```python
from build123d import *

# Parameters (mm, degrees)
SKETCH_W        = 54.3
SKETCH_H        = 39
PAD_DEPTH       = 2
SKETCH001_W     = 54.3
SKETCH001_H     = 2
PAD001_DEPTH    = 22
SKETCH003_W     = 6.85
SKETCH003_H     = 15
PAD003_DEPTH    = 22
SKETCH004_R     = 1.5
POCKET_DEPTH    = 15
SKETCH005_W     = 6.85
SKETCH005_H     = 15
PAD004_DEPTH    = 22
SKETCH006_R     = 1.5
POCKET001_DEPTH = 15
SKETCH007_W     = 25
SKETCH007_H     = 2
PAD005_DEPTH    = 22
POCKET002_DEPTH = 2.5
POCKET003_DEPTH = 5
FILLET_R        = 3
FILLET001_R     = 3
FILLET002_R     = 3
FILLET003_R     = 3
FILLET004_R     = 3
SKETCH010_R     = 1.786385
POCKET004_DEPTH = 5


with BuildPart() as part:
    # Sketch → Pad (new body)
    with BuildSketch(Plane.XY):
        with Locations((27.15, 21.5)):
            Rectangle(SKETCH_W, SKETCH_H)
    extrude(amount=PAD_DEPTH)

    # Sketch001 → Pad001 (join)
    with BuildSketch(Plane.XY):
        with Locations((27.15, 1)):
            Rectangle(SKETCH001_W, SKETCH001_H)
    extrude(amount=PAD001_DEPTH)

    # Sketch003 → Pad003 (join)
    with BuildSketch(Plane.XY):
        with Locations((3.425, 20.3)):
            Rectangle(SKETCH003_W, SKETCH003_H)
    extrude(amount=PAD003_DEPTH)

    # Sketch004 (on Face14 of Pad003) → Pocket (cut)
    with BuildSketch(Plane(origin=(0, 27.8, 0), x_dir=(-1, 0, 0), z_dir=(0, 1, 0))):
        with Locations((-3, 17)):
            Circle(SKETCH004_R)
        with Locations((-3, 7)):
            Circle(SKETCH004_R)
    extrude(amount=-POCKET_DEPTH, mode=Mode.SUBTRACT)

    # Sketch005 → Pad004 (join)
    with BuildSketch(Plane.XY):
        with Locations((50.875, 20.3)):
            Rectangle(SKETCH005_W, SKETCH005_H)
    extrude(amount=PAD004_DEPTH)

    # Sketch006 (on Face13 of Pad004) → Pocket001 (cut)
    with BuildSketch(Plane(origin=(0, 27.8, 0), x_dir=(-1, 0, 0), z_dir=(0, 1, 0))):
        with Locations((-51.3, 17)):
            Circle(SKETCH006_R)
        with Locations((-51.3, 7)):
            Circle(SKETCH006_R)
    extrude(amount=-POCKET001_DEPTH, mode=Mode.SUBTRACT)

    # Sketch007 (on Face4 of Pocket001) → Pad005 (join)
    with BuildSketch(Plane(origin=(0, 0, 0), x_dir=(1, 0, 0), z_dir=(0, 0, -1))):
        with Locations((12.5, -42)):
            Rectangle(SKETCH007_W, SKETCH007_H)
    extrude(amount=-PAD005_DEPTH)

    # Sketch008 (on Face18 of Pad005) → Pocket002 (cut)
    with BuildSketch(Plane(origin=(0, 2, 0), x_dir=(-1, 0, 0), z_dir=(0, 1, 0))):
        Polygon((-34.1, 12), (-35.675, 14.72798), (-38.825, 14.72798), (-40.4, 12), (-38.825, 9.27202), (-35.675, 9.27202), align=None)
        Polygon((-15.475, 14.72798), (-18.625, 14.72798), (-20.2, 12), (-18.625, 9.27202), (-15.475, 9.27202), (-13.9, 12), align=None)
    extrude(amount=-POCKET002_DEPTH, mode=Mode.SUBTRACT)

    # Sketch009 (on Face22 of Pocket002) → Pocket003 (cut)
    with BuildSketch(Plane(origin=(0, 43, 0), x_dir=(-1, 0, 0), z_dir=(0, 1, 0))):
        Polygon((-13.9, 12), (-15.475, 14.72798), (-18.625, 14.72798), (-20.2, 12), (-18.625, 9.27202), (-15.475, 9.27202), align=None)
    extrude(amount=-POCKET003_DEPTH, mode=Mode.SUBTRACT)

    # Fillet
    fillet_edges = [part.edges().sort_by_distance(p)[0] for p in [
        (0, 42, 22),
    ]]
    fillet(fillet_edges, radius=FILLET_R)

    # Fillet001
    fillet001_edges = [part.edges().sort_by_distance(p)[0] for p in [
        (0, 1, 22),
    ]]
    fillet(fillet001_edges, radius=FILLET001_R)

    # Fillet002
    fillet002_edges = [part.edges().sort_by_distance(p)[0] for p in [
        (0, 20.3, 22),
    ]]
    fillet(fillet002_edges, radius=FILLET002_R)

    # Fillet003
    fillet003_edges = [part.edges().sort_by_distance(p)[0] for p in [
        (54.3, 1, 22),
    ]]
    fillet(fillet003_edges, radius=FILLET003_R)

    # Fillet004
    fillet004_edges = [part.edges().sort_by_distance(p)[0] for p in [
        (54.3, 20.3, 22),
    ]]
    fillet(fillet004_edges, radius=FILLET004_R)

    # Sketch010 (on Face56 of Fillet004) → Pocket004 (cut)
    with BuildSketch(Plane(origin=(0, 43, 0), x_dir=(-1, 0, 0), z_dir=(0, 1, 0))):
        with Locations((-3, 17)):
            Circle(SKETCH010_R)
    extrude(amount=-POCKET004_DEPTH, mode=Mode.SUBTRACT)


solid = part.part
```
Geometry check sheet. Reference: the model listing, model coordinates, mm. A direction names the side the tool comes from. Coordinates: 2 decimals unless noted, no trailing zeros. Loops run counter-clockwise (first coordinate to the right, second up) from the corner with the lowest first, then second, coordinate; pieces in that order, holes last. Notation, with made-up numbers: (33, 39.5) -> (46, 39.5) arc R24 cw to (46, 67.5) -> close; hole circle Ø11 at (26.5, -17). An arc over 180 degrees is marked (long way). Put each result on its own line as item: value.
1) Cross-section at C-C on x = 23. Record the boundary of the cut face in (y, z), plus the area to 3 significant figures.
Result set:
outline: (0, 0) -> (43, 0) -> (43, 22) -> (41, 22) -> (41, 2) -> (2, 2) -> (2, 22) -> (0, 22) -> close
area: 166 mm^2
2) Tool access check on faces 1 (the flat face through (39.624, 1.014, 10.655)), 2 (the cylindrical face through (2.31, 20.4, 5.67)), 3 (the cylindrical face through (3.195, 20.405, 18.487)). Record the directions out of +Z, -Z, +X, -X, +Y, -Y that give a thin tool (end or side, any length) a straight path to the whole face; none if there is none.
Result set:
face 1: +Y, -Y
face 2: none
face 3: +Y
3) Release check for a two-part mould opening along Z. For faces 4 (the flat face through (19.401, 1.014, 13.383)), 5 (the flat face through (27, 22, 2)), 6 (the flat face through (12, 41, 12)) record: released by +Z, released by -Z, zero draft, split by the parting line, or undercut.
Result set:
face 4: undercut
face 5: released by +Z
face 6: zero draft
4) Thickness scan on line 1 (Z direction, x = 3, y = 24); line 2 (Y direction, x = 5.5, z = 10.75); line 3 (X direction, y = 16, z = 9.5). Record the ranges inside material, lowest first.
Result set:
line 1: z = 0 to 5.5, 8.5 to 15.5, 18.5 to 22
line 2: y = 0 to 2, 12.8 to 27.8, 41 to 43
line 3: x = 0 to 6.85, 47.45 to 54.3
5) Cross-section at A-A on z = 17. Record the boundary of the cut face in (x, y).
Result set:
outline: (0, 0) -> (54.3, 0) -> (54.3, 2) -> (0, 2) -> close; (0, 12.8) -> (1.5, 12.8) -> (1.5, 27.8) -> (0, 27.8) -> close; (0, 41) -> (1.21, 41) -> (1.21, 43) -> (0, 43) -> close; (4.5, 12.8) -> (6.85, 12.8) -> (6.85, 27.8) -> (4.5, 27.8) -> close; (4.79, 41) -> (25, 41) -> (25, 43) -> (4.79, 43) -> close; (47.45, 12.8) -> (49.8, 12.8) -> (49.8, 27.8) -> (47.45, 27.8) -> close; (52.8, 12.8) -> (54.3, 12.8) -> (54.3, 27.8) -> (52.8, 27.8) -> close
6) Cross-section at D-D on y = 3. Record the boundary of the cut face in (x, z).
Result set:
outline: (0, 0) -> (54.3, 0) -> (54.3, 2) -> (0, 2) -> close
7) Gauge pin test, flat ends, axial feed: pin 1 Ø4 at (y, z) = (38, 13) entering from +X; pin 2 Ø10 at (x, z) = (32, 11) entering from +Y; pin 3 Ø1.6 at (y, z) = (42, 15.5) entering from +X; pin 4 Ø5.5 at (x, z) = (50, 10.5) entering from +Y. Record the tip position at first contact, or that the pin passes through.
Result set:
pin 1: passes through
pin 2: stops at y = 2
pin 3: stops at x = 25
pin 4: stops at y = 27.8
8) Cross-section at B-B on z = 7. Record the boundary of the cut face in (x, y), plus the area to 3 significant figures.
Result set:
outline: (0, 0) -> (54.3, 0) -> (54.3, 2) -> (0, 2) -> close; (0, 12.8) -> (1.5, 12.8) -> (1.5, 27.8) -> (0, 27.8) -> close; (0, 41) -> (25, 41) -> (25, 43) -> (0, 43) -> close; (4.5, 12.8) -> (6.85, 12.8) -> (6.85, 27.8) -> (4.5, 27.8) -> close; (47.45, 12.8) -> (49.8, 12.8) -> (49.8, 27.8) -> (47.45, 27.8) -> close; (52.8, 12.8) -> (54.3, 12.8) -> (54.3, 27.8) -> (52.8, 27.8) -> close
area: 274 mm^2
